CAD build for the part. Positions are in the model's coordinates, mm. A direction names the side the tool comes from. Coordinates: 2 decimals unless noted, no trailing zeros. Write each loop counter-clockwise with the first axis right and the second up, starting at its lowest first coordinate (ties: lowest second). Pieces come first, ordered by that corner, then holes.
```python
from build123d import *

# Parameters (mm, degrees)
F0_W      = 100
F0_H      = 60
F1_DEPTH  = 18
F2_R      = 25
F3_DEPTH  = 12
F4_SIZE   = 5
F5_SIZE   = 2
F7_D      = 37
F9_DEPTH  = 60.001
F11_D     = 6
F13_D     = 3.3
F13_DEPTH = 10.1
F13_TIP   = 0.9914200214


with BuildPart() as f1:
    # F0 (on Top) → F1 (new body)
    with BuildSketch(Plane.XY):
        Rectangle(F0_W, F0_H)
    extrude(amount=F1_DEPTH)

    # F2 (on face) → F3 (join)
    with BuildSketch(Plane.XY.offset(18)):
        Circle(F2_R)
    extrude(amount=F3_DEPTH)

    # F4
    f4_edges = [f1.edges().sort_by_distance(p)[0] for p in [
        (50, -30, 9),
        (-50, -30, 9),
        (-50, 30, 9),
        (50, 30, 9),
    ]]
    chamfer(f4_edges, length=F4_SIZE)

    # F5
    f5_edges = [f1.edges().sort_by_distance(p)[0] for p in [
        (-25, 0, 30),
    ]]
    chamfer(f5_edges, length=F5_SIZE)

    # F7 (through all)
    with Locations(Plane.XY.offset(30)):
        with Locations((0, 0)):
            Hole(F7_D / 2)

    # F8 (on face) → F9 (cut, through all)
    with BuildSketch(Plane.XZ.offset(30)):
        with BuildLine():
            ThreePointArc((-10, 0), (0, -10), (10, 0))
            Line((10, 0), (-10, 0))
        make_face()
        with BuildLine():
            Line((-10, 0), (10, 0))
            ThreePointArc((10, 0), (0, 10), (-10, 0))
        make_face()
    extrude(amount=-F9_DEPTH, mode=Mode.SUBTRACT)

    # F11 (through all)
    with Locations(Plane.XY.offset(18)):
        with Locations((37.5, 0), (-37.5, 0)):
            Hole(F11_D / 2)

    # F13
    with Locations(Plane.XY.offset(18)):
        with Locations((35, 12), (-35, 12)):
            Hole(F13_D / 2, depth=F13_DEPTH)
            with Locations((0, 0, -(F13_DEPTH + F13_TIP / 2))):  # 118° drill point
                Cone(0, F13_D / 2, F13_TIP, mode=Mode.SUBTRACT)


solid = f1.part
```
Item 1: Flat gauge pins, fed straight in: pin 1 Ø12 at (y, z) = (21, 26) entering from +X; pin 2 Ø1.5 at (x, y) = (-33, 11) entering from +Z. Where does each tip first touch, or does it go through?
Item 2: Which spindle directions (+Z, -Z, +X, -X, +Y, -Y) get a long thin tool onto all of the face, cutting with end or side? Do faces 1 (the flat face through (30, 0, 0)), 2 (the cylindrical face through (36.31, 11, 12.88)). Say none if no direction does.
Item 3: Wall check: line 1 along Y through (x, z) = (-35, 12); line 2 along X through (y, z) = (12, 13); line 3 along X through (y, z) = (1.5, 13). Give the ranges that are in metal, low to high.
Item 4: Saw through at B-B, the plane y = 0. Write the cut outline in (x, z), and give its area (3 significant figures).
Item 5: Saw through at D-D, the plane z = 20.5. Write the cut outline in (x, y), and give its area (3 significant figures).
Item 6: Two-plate mould, pull along Y, no slides. Class faces 3 (the cylindrical face through (23.846, 7.509, 22.93)), 4 (the flat face through (-1, -30, 11)), 5 (the flat face through (-47, 28, 9)), 6 (the cylindrical face through (-33.69, 11, 12.88)): +Y half, -Y half, draft (parallel to the pull), parting line (faces both ways), or undercut.
Item 7: Saw through at C-C, the plane z = 2. Write the cut outline in (x, y), and give its area (3 significant figures).
Item 8: Saw through at A-A, the plane x = 0. Write the cut outline in (y, z).
Working result:
1. pin 1: stops at x = 20
1. pin 2: stops at z = 18
2. face 1: -Z, +X, -X, +Y, -Y
2. face 2: +Z
3. line 1: y = -30 to -1.66, 1.66 to 10.35, 13.65 to 30
3. line 2: x = -50 to -36.65, -33.35 to -14.08, 14.08 to 33.35, 36.65 to 50
3. line 3: x = -50 to -40.1, -34.9 to -18.44, 18.44 to 34.9, 40.1 to 50
4. outline: (-50, 0) - (-40.5, 0) - (-40.5, 18) - (-50, 18) - close; (-34.5, 0) - (-18.5, 0) - (-18.5, 30) - (-23, 30) - (-25, 28) - (-25, 18) - (-34.5, 18) - close; (18.5, 0) - (34.5, 0) - (34.5, 18) - (25, 18) - (25, 28) - (23, 30) - (18.5, 30) - close; (40.5, 0) - (50, 0) - (50, 18) - (40.5, 18) - close
4. area: 1,070 mm2
5. outline: circle Ø50 at (0, 0); hole circle Ø37 at (0, 0)
5. area: 888 mm2
6. face 3: parting line
6. face 4: -Y half
6. face 5: +Y half
6. face 6: undercut
7. outline: (-50, -25) - (-45, -30) - (-9.8, -30) - (-9.8, -15.69) arc R18.5 cw to (-9.8, 15.69) - (-9.8, 30) - (-45, 30) - (-50, 25) - close; (9.8, -30) - (45, -30) - (50, -25) - (50, 25) - (45, 30) - (9.8, 30) - (9.8, 15.69) arc R18.5 cw to (9.8, -15.69) - close; hole circle Ø6 at (-37.5, 0); hole circle Ø6 at (37.5, 0)
7. area: 4,330 mm2
8. outline: (-30, 10) - (-18.5, 10) - (-18.5, 30) - (-23, 30) - (-25, 28) - (-25, 18) - (-30, 18) - close; (18.5, 10) - (30, 10) - (30, 18) - (25, 18) - (25, 28) - (23, 30) - (18.5, 30) - close
